Source: CAD feature listing. Evaluate the final solid. Frame: model axes, mm. Coordinates: 2 decimals unless noted, no trailing zeros. Write each loop counter-clockwise with the first axis right and the second up, starting at its lowest first coordinate (ties: lowest second). Pieces come first, ordered by that corner, then holes. Notation, with made-up numbers: (10, -4) - (43, -4) arc R13 ccw to (43, 5) - close; hole circle Ø2 at (50, -17). An arc over 180 degrees is marked (long way). One line per question, with ' | ' between items.
from build123d import *

# Parameters (mm, degrees)
CROQUIS1_R              = 1.45
CROQUIS1_R_2            = 0.57
SALIENTE_EXTRUIR1_DEPTH = 1.5
CROQUIS2_R              = 0.57
CORTAR_EXTRUIR1_DEPTH   = 10


with BuildPart() as part:
    # Croquis1 → Saliente-Extruir1 (new body)
    with BuildSketch(Plane.XY):
        with BuildLine():
            Line((28.62, -15.24), (-28.62, -15.24))
            ThreePointArc((-28.62, -15.24), (-31.731269837, -13.951269837), (-33.02, -10.84))
            Line((-33.02, -10.84), (-33.02, 10.84))
            ThreePointArc((-33.02, 10.84), (-31.731269837, 13.951269837), (-28.62, 15.24))
            Line((-28.62, 15.24), (28.62, 15.24))
            ThreePointArc((28.62, 15.24), (31.731269837, 13.951269837), (33.02, 10.84))
            Line((33.02, 10.84), (33.02, -10.84))
            ThreePointArc((33.02, -10.84), (31.731269837, -13.951269837), (28.62, -15.24))
        make_face()
        with Locations((-28.62, 10.84)):
            Circle(CROQUIS1_R, mode=Mode.SUBTRACT)
        with Locations(Location((28.62, 10.84, 0), (0, 0, 180))):
            Circle(CROQUIS1_R, mode=Mode.SUBTRACT)
        with Locations((28.62, -10.84)):
            Circle(CROQUIS1_R, mode=Mode.SUBTRACT)
        with Locations(Location((-28.62, -10.84, 0), (0, 0, 180))):
            Circle(CROQUIS1_R, mode=Mode.SUBTRACT)
        with Locations((-24.13, -9.57)):
            Circle(CROQUIS1_R_2, mode=Mode.SUBTRACT)
        with Locations((-24.13, -12.11)):
            Circle(CROQUIS1_R_2, mode=Mode.SUBTRACT)
        with Locations((-21.59, -9.57)):
            Circle(CROQUIS1_R_2, mode=Mode.SUBTRACT)
        with Locations((-21.59, -12.11)):
            Circle(CROQUIS1_R_2, mode=Mode.SUBTRACT)
        with Locations((-19.05, -9.57)):
            Circle(CROQUIS1_R_2, mode=Mode.SUBTRACT)
        with Locations((-19.05, -12.11)):
            Circle(CROQUIS1_R_2, mode=Mode.SUBTRACT)
        with Locations((-16.51, -9.57)):
            Circle(CROQUIS1_R_2, mode=Mode.SUBTRACT)
        with Locations((-16.51, -12.11)):
            Circle(CROQUIS1_R_2, mode=Mode.SUBTRACT)
        with Locations((-13.97, -9.57)):
            Circle(CROQUIS1_R_2, mode=Mode.SUBTRACT)
        with Locations((-13.97, -12.11)):
            Circle(CROQUIS1_R_2, mode=Mode.SUBTRACT)
        with Locations((-11.43, -9.57)):
            Circle(CROQUIS1_R_2, mode=Mode.SUBTRACT)
        with Locations((-11.43, -12.11)):
            Circle(CROQUIS1_R_2, mode=Mode.SUBTRACT)
        with Locations((-8.89, -9.57)):
            Circle(CROQUIS1_R_2, mode=Mode.SUBTRACT)
        with Locations((-8.89, -12.11)):
            Circle(CROQUIS1_R_2, mode=Mode.SUBTRACT)
        with Locations((-6.35, -9.57)):
            Circle(CROQUIS1_R_2, mode=Mode.SUBTRACT)
        with Locations((-6.35, -12.11)):
            Circle(CROQUIS1_R_2, mode=Mode.SUBTRACT)
        with Locations((-3.81, -9.57)):
            Circle(CROQUIS1_R_2, mode=Mode.SUBTRACT)
        with Locations((-3.81, -12.11)):
            Circle(CROQUIS1_R_2, mode=Mode.SUBTRACT)
        with Locations((-1.27, -9.57)):
            Circle(CROQUIS1_R_2, mode=Mode.SUBTRACT)
        with Locations((-1.27, -12.11)):
            Circle(CROQUIS1_R_2, mode=Mode.SUBTRACT)
        with Locations((1.27, -9.57)):
            Circle(CROQUIS1_R_2, mode=Mode.SUBTRACT)
        with Locations((1.27, -12.11)):
            Circle(CROQUIS1_R_2, mode=Mode.SUBTRACT)
        with Locations((3.81, -9.57)):
            Circle(CROQUIS1_R_2, mode=Mode.SUBTRACT)
        with Locations((3.81, -12.11)):
            Circle(CROQUIS1_R_2, mode=Mode.SUBTRACT)
        with Locations((6.35, -9.57)):
            Circle(CROQUIS1_R_2, mode=Mode.SUBTRACT)
        with Locations((6.35, -12.11)):
            Circle(CROQUIS1_R_2, mode=Mode.SUBTRACT)
        with Locations((8.89, -9.57)):
            Circle(CROQUIS1_R_2, mode=Mode.SUBTRACT)
        with Locations((8.89, -12.11)):
            Circle(CROQUIS1_R_2, mode=Mode.SUBTRACT)
        with Locations((11.43, -9.57)):
            Circle(CROQUIS1_R_2, mode=Mode.SUBTRACT)
        with Locations((11.43, -12.11)):
            Circle(CROQUIS1_R_2, mode=Mode.SUBTRACT)
        with Locations((13.97, -9.57)):
            Circle(CROQUIS1_R_2, mode=Mode.SUBTRACT)
        with Locations((13.97, -12.11)):
            Circle(CROQUIS1_R_2, mode=Mode.SUBTRACT)
        with Locations((16.51, -9.57)):
            Circle(CROQUIS1_R_2, mode=Mode.SUBTRACT)
        with Locations((16.51, -12.11)):
            Circle(CROQUIS1_R_2, mode=Mode.SUBTRACT)
        with Locations((19.05, -9.57)):
            Circle(CROQUIS1_R_2, mode=Mode.SUBTRACT)
        with Locations((19.05, -12.11)):
            Circle(CROQUIS1_R_2, mode=Mode.SUBTRACT)
        with Locations((21.59, -9.57)):
            Circle(CROQUIS1_R_2, mode=Mode.SUBTRACT)
        with Locations((21.59, -12.11)):
            Circle(CROQUIS1_R_2, mode=Mode.SUBTRACT)
        with Locations((24.13, -9.57)):
            Circle(CROQUIS1_R_2, mode=Mode.SUBTRACT)
        with Locations((24.13, -12.11)):
            Circle(CROQUIS1_R_2, mode=Mode.SUBTRACT)
    extrude(amount=SALIENTE_EXTRUIR1_DEPTH)

    # Croquis2 → Cortar-Extruir1 (cut)
    with BuildSketch(Plane(origin=(0, 0, 0), x_dir=(-1, 0, 0), z_dir=(0, 0, -1))):
        with Locations((-30.48, -6.04)):
            Circle(CROQUIS2_R)
        with Locations((-27.94, -6.04)):
            Circle(CROQUIS2_R)
        with Locations((-25.4, -6.04)):
            Circle(CROQUIS2_R)
        with Locations((-22.86, -6.04)):
            Circle(CROQUIS2_R)
        with Locations((-20.32, -6.04)):
            Circle(CROQUIS2_R)
        with Locations((-17.78, -6.04)):
            Circle(CROQUIS2_R)
        with Locations((-15.24, -6.04)):
            Circle(CROQUIS2_R)
        with Locations((-12.7, -6.04)):
            Circle(CROQUIS2_R)
        with Locations((-10.16, -6.04)):
            Circle(CROQUIS2_R)
        with Locations((-7.62, -6.04)):
            Circle(CROQUIS2_R)
        with Locations((-5.08, -6.04)):
            Circle(CROQUIS2_R)
        with Locations((-2.54, -6.04)):
            Circle(CROQUIS2_R)
        with Locations((0, -6.04)):
            Circle(CROQUIS2_R)
        with Locations((2.54, -6.04)):
            Circle(CROQUIS2_R)
        with Locations((5.08, -6.04)):
            Circle(CROQUIS2_R)
        with Locations((7.62, -6.04)):
            Circle(CROQUIS2_R)
        with Locations((10.16, -6.04)):
            Circle(CROQUIS2_R)
        with Locations((12.7, -6.04)):
            Circle(CROQUIS2_R)
        with Locations((15.24, -6.04)):
            Circle(CROQUIS2_R)
        with Locations((17.78, -6.04)):
            Circle(CROQUIS2_R)
        with Locations((20.32, -6.04)):
            Circle(CROQUIS2_R)
        with Locations((22.86, -6.04)):
            Circle(CROQUIS2_R)
        with Locations((25.4, -6.04)):
            Circle(CROQUIS2_R)
        with Locations((27.94, -6.04)):
            Circle(CROQUIS2_R)
        with Locations((30.48, -6.04)):
            Circle(CROQUIS2_R)
        with Locations(Location((-5.08, 14.28, 0), (0, 0, 180))):
            Circle(CROQUIS2_R)
        with Locations(Location((-25.4, 14.28, 0), (0, 0, 180))):
            Circle(CROQUIS2_R)
        with Locations(Location((-5.08, 11.74, 0), (0, 0, 180))):
            Circle(CROQUIS2_R)
        with Locations(Location((-25.4, 11.74, 0), (0, 0, 180))):
            Circle(CROQUIS2_R)
        with Locations(Location((-5.08, 9.2, 0), (0, 0, 180))):
            Circle(CROQUIS2_R)
        with Locations(Location((-25.4, 9.2, 0), (0, 0, 180))):
            Circle(CROQUIS2_R)
        with Locations(Location((-5.08, 6.66, 0), (0, 0, 180))):
            Circle(CROQUIS2_R)
        with Locations(Location((-25.4, 6.66, 0), (0, 0, 180))):
            Circle(CROQUIS2_R)
        with Locations(Location((-5.08, 4.12, 0), (0, 0, 180))):
            Circle(CROQUIS2_R)
        with Locations(Location((-25.4, 4.12, 0), (0, 0, 180))):
            Circle(CROQUIS2_R)
        with Locations(Location((-15.24, -3.5, 0), (0, 0, 180))):
            Circle(CROQUIS2_R)
        with Locations(Location((-17.78, -3.5, 0), (0, 0, 180))):
            Circle(CROQUIS2_R)
        with Locations(Location((-20.32, -3.5, 0), (0, 0, 180))):
            Circle(CROQUIS2_R)
    extrude(amount=-CORTAR_EXTRUIR1_DEPTH, mode=Mode.SUBTRACT)


solid = part.part
Item 1: Ray query, line 1 along Y through (x, z) = (13.97, 0.5); line 2 along Y through (x, z) = (-9, 0.3); line 3 along Y through (x, z) = (-2.54, 0.65). Return the intervals inside material, ascending. Write a range as [from, to].
Check sheet entries:
line 1: [-15.24, -12.68], [-11.54, -10.14], [-9, 15.24] | line 2: [-15.24, -12.67], [-11.55, -10.13], [-9.01, 15.24] | line 3: [-15.24, -6.61], [-5.47, 15.24]
Item 2: Cut plane B-B on y = 13. Return loops of the section in (x, z), and give its area (3 significant figures).
Check sheet entries:
outline: (-32.45, 0) - (32.45, 0) - (32.45, 1.5) - (-32.45, 1.5) - close | area: 97.4 mm²
Item 3: Cut plane A-A on z = 0.9. State how many separate pieces and enclosed holes the cut face has, and give its area (3 significant figures).
Check sheet entries:
separate pieces: 1 | enclosed holes: 82 | area: 1,890 mm²
Item 4: Mould query, pull axis Y, two halves, no side actions, for faces 1 (the face through (-18.787, -12.616, 0.74)), 2 (the face through (33.02, 0, 1)). Classes: pulls with the +Y half, pulls with the -Y half, needs draft (parallel to the pull), parting line crosses it, or undercut.
Check sheet entries:
face 1: undercut | face 2: needs draft
Item 5: Pin query (flat end, axial travel): pin 1 Ø12 at (x, y) = (22.5, 0) entering from -Z. Return the tip coordinate at first contact, or that it passes through.
Check sheet entries:
pin 1: z = 0
